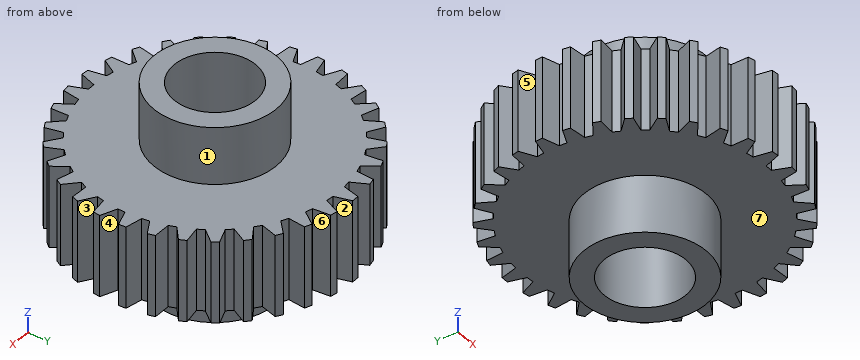
from build123d import *

# Parameters (mm, degrees)
BOSS_EXTRUDE1_DEPTH     = 5
SKETCH2_R               = 7.5
BOSS_EXTRUDE2_DEPTH     = 7
SKETCH3_R               = 5
CUT_EXTRUDE1_DEPTH      = 1
CUT_EXTRUDE1_DEPTH_BACK = 25


with BuildPart() as part:
    # Sketch1 → Boss-Extrude1 (new body, symmetric)
    with BuildSketch(Plane.XY):
        with BuildLine():
            Line((-1.102638188, 14.959418071), (-0.56896822, 16.990476013))
            Line((-0.56896822, 16.990476013), (0.299469927, 16.997362082))
            Line((0.299469927, 16.997362082), (0.865280327, 14.975022202))
            ThreePointArc((0.865280327, 14.975022202), (1.307399264, 14.942914949), (1.748376405, 14.897757548))
            Line((1.748376405, 14.897757548), (2.656782505, 16.791113921))
            Line((2.656782505, 16.791113921), (3.51083004, 16.63352255))
            Line((3.51083004, 16.63352255), (3.68368517, 14.540648664))
            ThreePointArc((3.68368517, 14.540648664), (4.111738104, 14.425450071), (4.53620012, 14.29765325))
            Line((4.53620012, 14.29765325), (5.786510188, 15.984877223))
            Line((5.786510188, 15.984877223), (6.595299608, 15.668504175))
            Line((6.595299608, 15.668504175), (6.368952034, 13.580738198))
            ThreePointArc((6.368952034, 13.580738198), (6.767468017, 13.386611843), (7.160073744, 13.180794513))
            Line((7.160073744, 13.180794513), (8.707098316, 14.600905414))
            Line((8.707098316, 14.600905414), (9.441397865, 14.137185235))
            Line((9.441397865, 14.137185235), (8.824028377, 12.129984469))
            ThreePointArc((8.824028377, 12.129984469), (9.178604003, 11.863946585), (9.525163646, 11.587547519))
            Line((9.525163646, 11.587547519), (11.312989225, 12.689218841))
            Line((11.312989225, 12.689218841), (11.946259403, 12.094911586))
            Line((11.946259403, 12.094911586), (10.960181343, 10.240821497))
            ThreePointArc((10.960181343, 10.240821497), (11.258001325, 9.912487385), (11.545989318, 9.575496367))
            Line((11.545989318, 9.575496367), (13.509999227, 10.318910838))
            Line((13.509999227, 10.318910838), (14.019352001, 9.61549632))
            Line((14.019352001, 9.61549632), (12.7002048, 7.981528553))
            ThreePointArc((12.7002048, 7.981528553), (12.930505147, 7.602765065), (13.149512852, 7.217361828))
            Line((13.149512852, 7.217361828), (15.218722658, 7.575650511))
            Line((15.218722658, 7.575650511), (15.58574869, 6.788551963))
            Line((15.58574869, 6.788551963), (13.981209764, 5.433762373))
            ThreePointArc((13.981209764, 5.433762373), (14.135666823, 5.018259007), (14.277778731, 4.598373027))
            Line((14.277778731, 4.598373027), (16.377401799, 4.558586437))
            Line((16.377401799, 4.558586437), (16.588835814, 3.716251652))
            Line((16.588835814, 3.716251652), (14.756897381, 2.689605862))
            ThreePointArc((14.756897381, 2.689605862), (14.82992867, 2.252379993), (14.890008487, 1.813187044))
            Line((14.890008487, 1.813187044), (16.944158969, 1.376763172))
            Line((16.944158969, 1.376763172), (16.992359189, 0.509636323))
            Line((16.992359189, 0.509636323), (14.999232277, -0.151760012))
            ThreePointArc((14.999232277, -0.151760012), (14.988198256, -0.594905903), (14.96407454, -1.037532242))
            Line((14.96407454, -1.037532242), (16.898510086, -1.854819902))
            Line((16.898510086, -1.854819902), (16.78173443, -2.715398591))
            Line((16.78173443, -2.715398591), (14.699455839, -2.987640883))
            ThreePointArc((14.699455839, -2.987640883), (14.604755306, -3.420690349), (14.497299951, -3.85075241))
            Line((14.497299951, -3.85075241), (16.24210502, -5.019364952))
            Line((16.24210502, -5.019364952), (15.964574065, -5.842291924))
            Line((15.964574065, -5.842291924), (13.868402767, -5.715540629))
            ThreePointArc((13.868402767, -5.715540629), (13.693458446, -6.122842133), (13.506555169, -6.524796354))
            Line((13.506555169, -6.524796354), (14.99866796, -8.002497074))
            Line((14.99866796, -8.002497074), (14.570412397, -8.758029606))
            Line((14.570412397, -8.758029606), (12.536109486, -8.236865845))
            ThreePointArc((12.536109486, -8.236865845), (12.28724432, -8.60369845), (12.027648293, -8.963017156))
            Line((12.027648293, -8.963017156), (13.213139961, -10.696398102))
            Line((13.213139961, -10.696398102), (12.649638063, -11.357229278))
            Line((12.649638063, -11.357229278), (10.750728545, -10.460489269))
            ThreePointArc((10.750728545, -10.460489269), (10.436937171, -10.773594688), (10.114030869, -11.077291166))
            Line((10.114030869, -11.077291166), (10.950054658, -13.003703433))
            Line((10.950054658, -13.003703433), (10.271672851, -13.545949094))
            Line((10.271672851, -13.545949094), (8.576788264, -12.306043355))
            ThreePointArc((8.576788264, -12.306043355), (8.209411919, -12.554105143), (7.834866018, -12.791203011))
            Line((7.834866018, -12.791203011), (8.291205849, -14.841021042))
            Line((8.291205849, -14.841021042), (7.522462619, -15.245083015))
            Line((7.522462619, -15.245083015), (6.092860509, -13.706824972))
            ThreePointArc((6.092860509, -13.706824972), (5.68517713, -13.88087753), (5.272528696, -14.042807453))
            Line((5.272528696, -14.042807453), (5.332691259, -16.141945482))
            Line((5.332691259, -16.141945482), (4.501370988, -16.393219916))
            Line((4.501370988, -16.393219916), (3.3887209, -14.612206222))
            ThreePointArc((3.3887209, -14.612206222), (2.955465228, -14.705958836), (2.519628449, -14.786868244))
            Line((2.519628449, -14.786868244), (2.181439312, -16.859457955))
            Line((2.181439312, -16.859457955), (1.317588082, -16.948863137))
            Line((1.317588082, -16.948863137), (0.562104089, -14.989464266))
            ThreePointArc((0.562104089, -14.989464266), (0.118935112, -14.999528474), (-0.324337735, -14.996493091))
            Line((-0.324337735, -14.996493091), (-1.048655536, -16.96762569))
            Line((-1.048655536, -16.96762569), (-1.91381589, -16.891930285))
            Line((-1.91381589, -16.891930285), (-2.284828629, -14.824964018))
            ThreePointArc((-2.284828629, -14.824964018), (-2.721893629, -14.750976072), (-3.156581508, -14.664105605))
            Line((-3.156581508, -14.664105605), (-4.24084924, -16.462539225))
            Line((-4.24084924, -16.462539225), (-5.07604957, -16.22447906))
            Line((-5.07604957, -16.22447906), (-5.049181687, -14.124650944))
            ThreePointArc((-5.049181687, -14.124650944), (-5.464346042, -13.969284961), (-5.874738201, -13.801719134))
            Line((-5.874738201, -13.801719134), (-7.279767603, -15.362453699))
            Line((-7.279767603, -15.362453699), (-8.054821592, -14.97063289))
            Line((-8.054821592, -14.97063289), (-7.631044164, -12.913836183))
            ThreePointArc((-7.631044164, -12.913836183), (-8.009302753, -12.682707496), (-8.380566549, -12.440502575))
            Line((-8.380566549, -12.440502575), (-10.055576198, -13.70712907))
            Line((-10.055576198, -13.70712907), (-10.742471376, -13.175709041))
            Line((-10.742471376, -13.175709041), (-9.937100822, -11.236281736))
            ThreePointArc((-9.937100822, -11.236281736), (-10.264782393, -10.937743936), (-10.583499387, -10.629653839))
            Line((-10.583499387, -10.629653839), (-12.467950069, -11.556393082))
            Line((-12.467950069, -11.556393082), (-13.041860255, -10.904580739))
            Line((-13.041860255, -10.904580739), (-11.884004765, -9.152618792))
            ThreePointArc((-11.884004765, -9.152618792), (-12.149266054, -8.797461813), (-12.403916981, -8.434621718))
            Line((-12.403916981, -8.434621718), (-14.42969974, -8.987978939))
            Line((-14.42969974, -8.987978939), (-14.869882324, -8.239332477))
            Line((-14.869882324, -8.239332477), (-13.401389813, -6.738156357))
            ThreePointArc((-13.401389813, -6.738156357), (-13.594643584, -6.339216499), (-13.776024698, -5.934740391))
            Line((-13.776024698, -5.934740391), (-15.869922466, -6.094715819))
            Line((-15.869922466, -6.094715819), (-16.160468103, -5.276293272))
            Line((-16.160468103, -5.276293272), (-14.434413716, -4.080159395))
            ThreePointArc((-14.434413716, -4.080159395), (-14.548675275, -3.651855384), (-14.650230989, -3.220362085))
            Line((-14.650230989, -3.220362085), (-16.736564846, -2.98117379))
            Line((-16.736564846, -2.98117379), (-16.866972459, -2.122555081))
            Line((-16.866972459, -2.122555081), (-14.945740298, -1.274694842))
            ThreePointArc((-14.945740298, -1.274694842), (-14.976879935, -0.8325067), (-14.994939762, -0.389591502))
            Line((-14.994939762, -0.389591502), (-16.998304165, 0.240115627))
            Line((-16.998304165, 0.240115627), (-16.963860484, 1.107897781))
            Line((-16.963860484, 1.107897781), (-14.916888886, 1.576840503))
            ThreePointArc((-14.916888886, 1.576840503), (-14.863781133, 2.016930945), (-14.797692342, 2.455259933))
            Line((-14.797692342, 2.455259933), (-16.645680483, 3.45272664))
            Line((-16.645680483, 3.45272664), (-16.447630392, 4.29830833))
            Line((-16.447630392, 4.29830833), (-14.348902243, 4.371384725))
            ThreePointArc((-14.348902243, 4.371384725), (-14.213466553, 4.793471451), (-14.065617767, 5.211371877))
            Line((-14.065617767, 5.211371877), (-15.691438539, 6.540547117))
            Line((-15.691438539, 6.540547117), (-15.336940083, 7.333366818))
            Line((-15.336940083, 7.333366818), (-13.262308888, 7.007935713))
            ThreePointArc((-13.262308888, 7.007935713), (-13.049440259, 7.396763409), (-12.825175117, 7.779131264))
            Line((-12.825175117, 7.779131264), (-14.170067122, 9.391975179))
            Line((-14.170067122, 9.391975179), (-13.6719328, 10.103378321))
            Line((-13.6719328, 10.103378321), (-11.696381135, 9.391201645))
            ThreePointArc((-11.696381135, 9.391201645), (-11.413773194, 9.732717065), (-11.121197223, 10.065732577))
            Line((-11.121197223, 10.065732577), (-12.136552559, 11.903952788))
            Line((-12.136552559, 11.903952788), (-11.512786244, 12.508227408))
            Line((-11.512786244, 12.508227408), (-9.707715693, 11.435045082))
            ThreePointArc((-9.707715693, 11.435045082), (-9.365582628, 11.716904968), (-9.015270286, 11.98853209))
            Line((-9.015270286, 11.98853209), (-9.664391366, 13.985690527))
            Line((-9.664391366, 13.985690527), (-8.937537597, 14.460996567))
            Line((-8.937537597, 14.460996567), (-7.368188113, 13.065596195))
            ThreePointArc((-7.368188113, 13.065596195), (-6.978895504, 13.277613398), (-6.583507991, 13.478034817))
            Line((-6.583507991, 13.478034817), (-6.842933888, 15.561948972))
            Line((-6.842933888, 15.561948972), (-6.039263054, 15.891107632))
            Line((-6.039263054, 15.891107632), (-4.762355017, 14.22392262))
            ThreePointArc((-4.762355017, 14.22392262), (-4.339972912, 14.358434285), (-3.913800564, 14.480406249))
            Line((-3.913800564, 14.480406249), (-3.774154951, 16.575758034))
            Line((-3.774154951, 16.575758034), (-2.92271381, 16.746872663))
            Line((-2.92271381, 16.746872663), (-1.984398002, 14.868159421))
            ThreePointArc((-1.984398002, 14.868159421), (-1.544192393, 14.920303946), (-1.102638188, 14.959418071))
        make_face()
    extrude(amount=BOSS_EXTRUDE1_DEPTH, both=True)

    # Sketch2 → Boss-Extrude2 (add)
    with BuildSketch(Plane.XY.offset(5)):
        Circle(SKETCH2_R)
    boss_extrude2 = extrude(amount=BOSS_EXTRUDE2_DEPTH)

    # Mirror1: Boss-Extrude2 across plane
    add(boss_extrude2.mirror(Plane.XY))

    # Sketch3 → Cut-Extrude1 (cut, two sides)
    with BuildSketch(Plane.XY.offset(12)) as cut_extrude1_sk:
        Circle(SKETCH3_R)
    extrude(amount=CUT_EXTRUDE1_DEPTH, mode=Mode.SUBTRACT)
    extrude(cut_extrude1_sk.sketch, amount=-CUT_EXTRUDE1_DEPTH_BACK, mode=Mode.SUBTRACT)


solid = part.part
Geometry: final body of the model. Coordinates: model frame, mm. Face numbers are marked on the shaded views. A direction names the side the tool comes from. Coordinates: 2 decimals unless noted, no trailing zeros. Loops run counter-clockwise (first coordinate to the right, second up) from the corner with the lowest first, then second, coordinate; pieces in that order, holes last. Notation, with made-up numbers: (78.25, -2) - (89.25, -2) arc R26 cw to (89.25, 25) - close; hole circle Ø7 at (42.5, 14.5). An arc over 180 degrees is marked (long way). Put each result on its own line as item: value. Start each with the question number.
Q1. Cut plane A-A, the plane y = 6. Return loops of the section in (x, z), and give its area (3 significant figures).
Q2. Line query: line 1 (Y direction, x = 0, z = -7); line 2 (Y direction, x = 0, z = 4.5); line 3 (Z direction, x = -6.5, y = -10.5). Output: solid intervals per line, ascending.
Q3. Pull-direction query (X, two-part tool) for the marked faces 1, 2 and 3; classes: released by +X, released by -X, zero draft, split by the parting line, or undercut.
Q4. Pin query (flat end, axial travel): pin 1 Ø8 at (x, y) = (-5, 12) entering from +Z; pin 2 Ø4 at (y, z) = (-5.5, 1) entering from +X; pin 3 Ø1.5 at (x, z) = (-9.5, 1.5) entering from -Y. Return the tip coordinate at first contact, or that it passes through.
Q5. Set-up query: the marked faces 4, 5, 6 and 7. Return all of +Z, -Z, +X, -X, +Y, -Y with unobstructed straight access to the full face (end or side cutting, diameter ignored); none if empty.
Filled sheet:
1. outline: (-15.03, -5) - (-4.5, -5) - (-4.5, -12) - (4.5, -12) - (4.5, -5) - (14.65, -5) - (14.65, 5) - (4.5, 5) - (4.5, 12) - (-4.5, 12) - (-4.5, 5) - (-15.03, 5) - close
1. area: 423 mm²
2. line 1: -7.5 to -5, 5 to 7.5
2. line 2: -15 to -5, 5 to 16.99
2. line 3: -5 to 5
3. face 1: split by the parting line
3. face 2: undercut
3. face 3: released by +X
4. pin 1: z = 5
4. pin 2: x = 16.24
4. pin 3: y = -13.71
5. face 4: +Z, -Z, +X
5. face 5: +Z, -Z, -X
5. face 6: +Z, -Z, +Y
5. face 7: -Z
